from build123d import *

# Parameters (mm, degrees)
F0_W     = 21.445978
F0_H     = 76.069072
F1_DEPTH = 12.7


with BuildPart() as f1:
    # F0 (on Front) → F1 (new body, symmetric)
    with BuildSketch(Plane.XZ):
        Polygon((21.445978, 35.285052), (49.674021, 35.285052), (49.674021, 47.749385), (0, 47.749385), (0, 35.285052), align=None)
        with Locations((10.722989, -2.749484)):
            Rectangle(F0_W, F0_H)
        Polygon((43.991752, -40.78402), (21.445978, -40.78402), (0, -40.78402), (0, -60.580309), (43.991752, -60.580309), align=None)
    extrude(amount=F1_DEPTH, both=True)


solid = f1.part
Can you work these out from the model? Positions are in its coordinate system, mm. A direction names the side the tool comes from. Give positions to 0.01 mm unless a question says otherwise; leave off trailing zeros. Write each loop counter-clockwise with the first axis right and the second up, starting at its lowest first coordinate (ties: lowest second). Pieces come first, ordered by that corner, then holes. Notation, with made-up numbers: (12, 25) -> (46, 25) arc R12 ccw to (46, 45) -> close; hole circle Ø11 at (-19.75, 80.5). An arc over 180 degrees is marked (long way). Answer as a JSON object with one key per item and string values. Group by question number.
Item 1: Suppose I cut it at C-C (z = 4.5). Please give me the cut outline in (x, y).
Item 2: For faces 4 (the face through (19, 12.7, -6)), 5 (the face through (35, 0, 35.285)), 6 (the face through (43.992, 0, -51)), which set-ups out of +Z, -Z, +X, -X, +Y, -Y let a thin tool reach every point of the face, with its end or its side?
Item 3: I'm going to push flat-ended pins straight in: P1, Ø6, axis at y = 2, z = -52, coming from the +X side; P2, Ø1, axis at y = 1, z = -21.5, coming from the +X side. Where does each tip first touch, or does it pass through?
Item 4: Suppose I cut it at D-D (z = -49.5). Please give me the cut outline in (x, y), plus the area to 3 significant figures.
Item 5: Suppose I cut it at A-A (x = 42). Please give me the cut outline in (y, z).
Item 6: We'd pull the mould along Z, two halves only. Please class faces 1 (the face through (33, 0, -40.784)), 2 (the face through (49.674, 0, 41)), 3 (the face through (22, 0, -60.58)): +Z half, -Z half, draft (parallel to the pull), parting line (faces both ways), or undercut.
Item 7: Suppose I cut it at B-B (y = 1.25). Please give me the cut outline in (x, z).
Item 8: Please list where these lines run through material, in increasing order: line 1 (Z direction, x = 33, y = 5); line 2 (X direction, y = 10.75, z = -2); line 3 (Z direction, x = 48, y = 11.25). Write a range as [from, to].
Findings:
{
 "1": {"outline": "(0, -12.7) -> (21.45, -12.7) -> (21.45, 12.7) -> (0, 12.7) -> close"},
 "2": {"face 4": "+Z, -Z, +X, -X, +Y", "face 5": "+X, +Y, -Y", "face 6": "-Z, +X, +Y, -Y"},
 "3": {"P1": "stops at x = 43.99", "P2": "stops at x = 21.45"},
 "4": {"outline": "(0, -12.7) -> (43.99, -12.7) -> (43.99, 12.7) -> (0, 12.7) -> close", "area": "1,120 mm²"},
 "5": {"outline": "(-12.7, -60.58) -> (12.7, -60.58) -> (12.7, -40.78) -> (-12.7, -40.78) -> close; (-12.7, 35.29) -> (12.7, 35.29) -> (12.7, 47.75) -> (-12.7, 47.75) -> close"},
 "6": {"face 1": "undercut", "face 2": "draft", "face 3": "-Z half"},
 "7": {"outline": "(0, -60.58) -> (43.99, -60.58) -> (43.99, -40.78) -> (21.45, -40.78) -> (21.45, 35.29) -> (49.67, 35.29) -> (49.67, 47.75) -> (0, 47.75) -> close"},
 "8": {"line 1": "z = [-60.58, -40.78], [35.29, 47.75]", "line 2": "x = [0, 21.45]", "line 3": "z = [35.29, 47.75]"}
}
